Read the model definition and answer for the solid it produces. Units are mm, in the model's axes. A direction names the side the tool comes from. Give positions to 0.01 mm unless a question says otherwise; leave off trailing zeros. Order: outer loops, then holes, each group sorted by start corner. A loop starts at its lowest first (then second) coordinate and runs counter-clockwise, first axis right, second up. Notation, with made-up numbers: (56.5, 60) - (93.5, 60) arc R28 cw to (93.5, 84) - close; hole circle Ø10 at (49, 65.5). An arc over 180 degrees is marked (long way). Write each question's results on one line, items separated by ' | '.
from build123d import *

# Parameters (mm, degrees)
BOSS_EXTRUDE1_DEPTH = 31.75
SKETCH2_R           = 3.175
CUT_EXTRUDE1_DEPTH  = 6.35
SKETCH4_R           = 3.175
CUT_EXTRUDE2_DEPTH  = 6.35


with BuildPart() as part:
    # Sketch1 → Boss-Extrude1 (new body)
    with BuildSketch(Plane(origin=(0, 0, 0), x_dir=(1, 0, 0), z_dir=(0, 1, 0))):
        Polygon((-22.225, 19.05), (22.225, 19.05), (47.625, 19.05), (47.625, 12.7), (22.225, 12.7), (22.225, -12.7), (47.625, -12.7), (47.625, -19.05), (25.4, -19.05), (25.4, -63.5), (19.05, -63.5), (19.05, -19.05), (-19.05, -19.05), (-19.05, -63.5), (-25.4, -63.5), (-25.4, -19.05), (-47.625, -19.05), (-47.625, -12.7), (-22.225, -12.7), (-22.225, 12.7), (-47.625, 12.7), (-47.625, 19.05), align=None)
    extrude(amount=BOSS_EXTRUDE1_DEPTH)

    # Sketch2 → Cut-Extrude1 (cut)
    with BuildSketch(Plane.XY.offset(19.05)):
        with Locations((34.925, 10.16)):
            Circle(SKETCH2_R)
        with Locations((-34.925, 10.16)):
            Circle(SKETCH2_R)
    cut_extrude1 = extrude(amount=-CUT_EXTRUDE1_DEPTH, mode=Mode.SUBTRACT)

    # Mirror1: Cut-Extrude1 across plane
    add(cut_extrude1.mirror(Plane.XY), mode=Mode.SUBTRACT)

    # Sketch4 → Cut-Extrude2 (cut)
    with BuildSketch(Plane.ZY.offset(25.4)):
        with Locations((40.823194714, 25.807528855)):
            Circle(SKETCH4_R)
        with Locations((57.15, 6.35)):
            Circle(SKETCH4_R)
    cut_extrude2 = extrude(amount=-CUT_EXTRUDE2_DEPTH, mode=Mode.SUBTRACT)

    # Mirror2: Cut-Extrude2 across plane
    add(cut_extrude2.mirror(Plane(origin=(0, 0, 0), x_dir=(0, 0, 1), z_dir=(1, 0, 0))), mode=Mode.SUBTRACT)


solid = part.part
(1) Section C-C (y = 24) is taken. Give the vertices of the cut face in (x, z) (3 decimals), plus the area to 3 significant figures.
Conclusion:
outline: (-47.625, -19.05) - (47.625, -19.05) - (47.625, -12.7) - (22.225, -12.7) - (22.225, 12.7) - (47.625, 12.7) - (47.625, 19.05) - (25.4, 19.05) - (25.4, 38.213) - (19.05, 38.213) - (19.05, 19.05) - (-19.05, 19.05) - (-19.05, 38.213) - (-25.4, 38.213) - (-25.4, 19.05) - (-47.625, 19.05) - (-47.625, 12.7) - (-22.225, 12.7) - (-22.225, -12.7) - (-47.625, -12.7) - close; (-25.4, 43.433) - (-19.05, 43.433) - (-19.05, 63.5) - (-25.4, 63.5) - close; (19.05, 43.433) - (25.4, 43.433) - (25.4, 63.5) - (19.05, 63.5) - close | area: 2,840 mm^2
(2) Each of these flat-tipped pins is pushed along its axis until it touches: pin 1 (1 mm diameter, centred on y = 5.5, z = 48.5, fed in from +X); pin 2 (7.5 mm diameter, centred on x = 29.5, y = 9, fed in from +Z); pin 3 (9.5 mm diameter, centred on y = 22, z = 34, fed in from -X); pin 4 (10 mm diameter, centred on x = 14.5, y = 26.5, fed in from +Z). Where does it stop, or does it pass through?
Conclusion:
pin 1: x = 25.4 | pin 2: z = 19.05 | pin 3: x = -25.4 | pin 4: z = 63.5
(3) For faces 5 (the face through (35, 16, 12.7)), 6 (the face through (19.05, 16, 42)), 7 (the face through (-22.27, 6.49, 53.98)), 8 (the face through (-35, 16, 12.7)), 9 (the face through (37, 16, 19.05)), determine the directions among +Z, -Z, +X, -X, +Y, -Y from which every point of the face is accessible in a straight line to the end or side of a thin tool.
Conclusion:
face 5: +X, +Y, -Y | face 6: +Z, +Y, -Y | face 7: +X, -X | face 8: -X, +Y, -Y | face 9: +Z, +X, +Y, -Y
(4) Section B-B (x = 42.5) is taken. Give the vertices of the cut face in (y, z), plus the area to 3 significant figures.
Conclusion:
outline: (0, -19.05) - (31.75, -19.05) - (31.75, -12.7) - (0, -12.7) - close; (0, 12.7) - (31.75, 12.7) - (31.75, 19.05) - (0, 19.05) - close | area: 403 mm^2
(5) Section D-D (z = 39) is taken. Give the vertices of the cut face in (x, y), plus the area to 3 significant figures.
Conclusion:
outline: (-25.4, 0) - (-19.05, 0) - (-19.05, 23.21) - (-25.4, 23.21) - close; (-25.4, 28.41) - (-19.05, 28.41) - (-19.05, 31.75) - (-25.4, 31.75) - close; (19.05, 0) - (25.4, 0) - (25.4, 23.21) - (19.05, 23.21) - close; (19.05, 28.41) - (25.4, 28.41) - (25.4, 31.75) - (19.05, 31.75) - close | area: 337 mm^2
(6) The mould has two halves that part along X. Classify faces 1 (the face through (-19.05, 16, 41)), 2 (the face through (-36, 16, 19.05)), 3 (the face through (0, 16, 19.05)), 4 (the face through (-47.625, 16, 16)): pulls with the +X half, pulls with the -X half, needs draft (parallel to the pull), parting line crosses it, or undercut.
Conclusion:
face 1: undercut | face 2: needs draft | face 3: undercut | face 4: pulls with the -X half
(7) Section A-A (z = 57.15) is taken. Give the vertices of the cut face in (x, y) (3 decimals), plus the area to 3 significant figures.
Conclusion:
outline: (-25.4, 0) - (-19.05, 0) - (-19.05, 3.175) - (-25.4, 3.175) - close; (-25.4, 9.525) - (-19.05, 9.525) - (-19.05, 31.75) - (-25.4, 31.75) - close; (19.05, 0) - (25.4, 0) - (25.4, 3.175) - (19.05, 3.175) - close; (19.05, 9.525) - (25.4, 9.525) - (25.4, 31.75) - (19.05, 31.75) - close | area: 323 mm^2
(8) Consider probe 1 along Z at (x, y) = (37, 7.5); probe 2 along X at (y, z) = (20, 27); probe 3 along Z at (x, y) = (-22, 6). Determine where each line is inside the solid, lowest interval first. Write a range as [from, to].
Conclusion:
probe 1: [-19.05, -12.7], [12.7, 19.05] | probe 2: [-25.4, -19.05], [19.05, 25.4] | probe 3: [-19.05, 53.99], [60.31, 63.5]
